The listing builds one solid part. Answer for the finished solid, in the listing's coordinates (mm). Face numbers are marked on the shaded views. A direction names the side the tool comes from. Give positions to 0.01 mm unless a question says otherwise; leave off trailing zeros. Write each loop counter-clockwise with the first axis right and the second up, starting at its lowest first coordinate (ties: lowest second). Pieces come first, ordered by that corner, then holes. Notation, with made-up numbers: M 28,24.5 L 82,24.5 A27 cw 82,52.5 Z; hole C -16,64.25 d11. An arc over 180 degrees is marked long. Return JSON: item names as keys, results as strings.
from build123d import *

# Parameters (mm, degrees)
SKETCH1_R           = 14
SKETCH1_R_2         = 1.6
SKETCH1_R_3         = 1.7
SKETCH1_R_4         = 2.95
BOSS_EXTRUDE1_DEPTH = 1
SKETCH1_3_R         = 2.95
BOSS_EXTRUDE2_DEPTH = 31


with BuildPart() as part:
    # Sketch1 → Boss-Extrude1 (new body)
    with BuildSketch(Plane(origin=(0, 0, 0), x_dir=(1, 0, 0), z_dir=(0, 1, 0))):
        with Locations(Location((0, 0, 0), (0, 0, 270))):
            Circle(SKETCH1_R)
        with Locations(Location((0, 10, 0), (0, 0, 270))):
            Circle(SKETCH1_R_2, mode=Mode.SUBTRACT)
        with Locations(Location((10, 0, 0), (0, 0, 270))):
            Circle(SKETCH1_R_2, mode=Mode.SUBTRACT)
        with Locations(Location((0, -10, 0), (0, 0, 270))):
            Circle(SKETCH1_R_2, mode=Mode.SUBTRACT)
        with Locations(Location((-10, 0, 0), (0, 0, 270))):
            Circle(SKETCH1_R_2, mode=Mode.SUBTRACT)
        with Locations(Location((-5.303300859, 5.303300859, 0), (0, 0, 270))):
            Circle(SKETCH1_R_3, mode=Mode.SUBTRACT)
        with Locations(Location((-5.303300859, -5.303300859, 0), (0, 0, 270))):
            Circle(SKETCH1_R_3, mode=Mode.SUBTRACT)
        with Locations(Location((5.303300859, 5.303300859, 0), (0, 0, 270))):
            Circle(SKETCH1_R_3, mode=Mode.SUBTRACT)
        with Locations(Location((5.303300859, -5.303300859, 0), (0, 0, 270))):
            Circle(SKETCH1_R_3, mode=Mode.SUBTRACT)
        with Locations(Location((0, 0, 0), (0, 0, 270))):
            Circle(SKETCH1_R_4, mode=Mode.SUBTRACT)
    extrude(amount=BOSS_EXTRUDE1_DEPTH)

    # Sketch1_3 → Boss-Extrude2 (add)
    with BuildSketch(Plane(origin=(0, 0, 0), x_dir=(1, 0, 0), z_dir=(0, 1, 0))):
        with Locations(Location((0, 0, 0), (0, 0, 270))):
            Circle(SKETCH1_3_R)
    extrude(amount=BOSS_EXTRUDE2_DEPTH)


solid = part.part
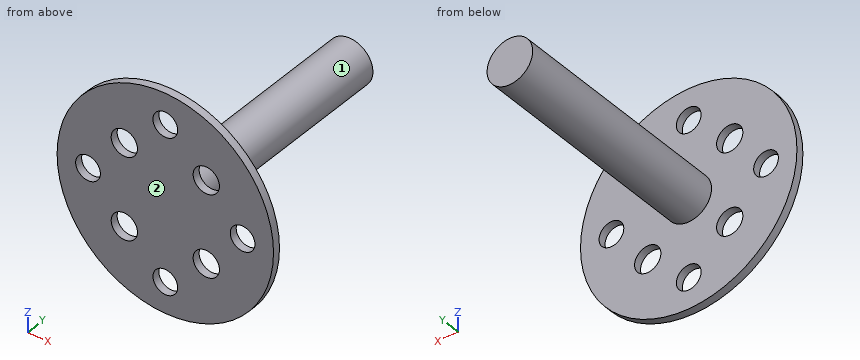
Item 1: Given pin 1 Ø6 at (x, z) = (-3.5, -5) entering from -Y; pin 2 Ø1.5 at (x, z) = (6.5, -2.5) entering from +Y; pin 3 Ø4 at (y, z) = (11, -2.5) entering from +X; pin 4 Ø6 at (x, y) = (1.5, 27.5) entering from +Z, each flat-ended and moving along its own axis, determine where each tip first touches the part or whether it passes through.
Geometry results:
{"pin 1": "stops at y = 0", "pin 2": "stops at y = 1", "pin 3": "stops at x = 2.91", "pin 4": "stops at z = 2.95"}
Item 2: A cutting plane is placed at A-A, the plane z = 0. Write down the section's boundary in (x, y), plus the area to 3 significant figures.
Geometry results:
{"outline": "M -14,0 L -11.6,0 L -11.6,1 L -14,1 Z; M -8.4,0 L 8.4,0 L 8.4,1 L 2.95,1 L 2.95,31 L -2.95,31 L -2.95,1 L -8.4,1 Z; M 11.6,0 L 14,0 L 14,1 L 11.6,1 Z", "area": "199 mm2"}
Item 3: Find the intervals of material crossed by line 1 (Y direction, x = -4.25, z = -11); line 2 (Z direction, x = -0.25, y = 12); line 3 (X direction, y = 16, z = -0.75), in increasing order.
Geometry results:
{"line 1": "y = 0 to 1", "line 2": "z = -2.94 to 2.94", "line 3": "x = -2.85 to 2.85"}
Item 4: A cutting plane is placed at C-C, the plane z = 10.5. Write down the section's boundary in (x, y), plus the area to 3 significant figures.
Geometry results:
{"outline": "M -9.26,0 L -1.52,0 L -1.52,1 L -9.26,1 Z; M 1.52,0 L 9.26,0 L 9.26,1 L 1.52,1 Z", "area": "15.5 mm2"}
Item 5: A cutting plane is placed at D-D, the plane x = -10. Write down the section's boundary in (y, z), plus the area to 3 significant figures.
Geometry results:
{"outline": "M 0,-9.8 L 1,-9.8 L 1,-1.6 L 0,-1.6 Z; M 0,1.6 L 1,1.6 L 1,9.8 L 0,9.8 Z", "area": "16.4 mm2"}
Item 6: A cutting plane is placed at B-B, the plane x = 0. Write down the section's boundary in (y, z).
Geometry results:
{"outline": "M 0,-14 L 1,-14 L 1,-11.6 L 0,-11.6 Z; M 0,-8.4 L 1,-8.4 L 1,-2.95 L 31,-2.95 L 31,2.95 L 1,2.95 L 1,8.4 L 0,8.4 Z; M 0,11.6 L 1,11.6 L 1,14 L 0,14 Z"}
Item 7: Which of the six approach directions +Z, -Z, +X, -X, +Y, -Y give full straight-line access (tool end or side, diameter ignored) to the marked faces 1 and 2?
Geometry results:
{"face 1": "+Y", "face 2": "+Z, -Z, +X, -X, -Y"}
